from build123d import *

# Parameters (mm, degrees)
F1_DEPTH = 25.4


with BuildPart() as f1:
    # F0 (on Top) → F1 (new body)
    with BuildSketch(Plane.XY):
        with BuildLine():
            Line((-308.69023, -16.839156), (-308.69023, -82.879156))
            Line((-308.69023, -82.879156), (265.34977, -82.879156))
            Line((265.34977, -82.879156), (265.34977, -16.839156))
            Line((265.34977, -16.839156), (43.73477, -16.839156))
            ThreePointArc((43.73477, -16.839156), (11.405848, -3.448078), (-1.98523, 28.880844))
            Line((-1.98523, 28.880844), (-1.98523, 414.960844))
            ThreePointArc((-1.98523, 414.960844), (11.405848, 447.289766), (43.73477, 460.680844))
            Line((43.73477, 460.680844), (265.34977, 460.680844))
            Line((265.34977, 460.680844), (265.34977, 526.720844))
            Line((265.34977, 526.720844), (-308.69023, 526.720844))
            Line((-308.69023, 526.720844), (-308.69023, 460.680844))
            Line((-308.69023, 460.680844), (-87.07523, 460.680844))
            ThreePointArc((-87.07523, 460.680844), (-54.746308, 447.289766), (-41.35523, 414.960844))
            Line((-41.35523, 414.960844), (-41.35523, 301.353365))
            Line((-41.35523, 301.353365), (-41.35523, 28.880844))
            ThreePointArc((-41.35523, 28.880844), (-54.746308, -3.448078), (-87.07523, -16.839156))
            Line((-87.07523, -16.839156), (-308.69023, -16.839156))
        make_face()
    extrude(amount=F1_DEPTH)


solid = f1.part
Can you work these out from the model? Positions are in its coordinate system, mm. A direction names the side the tool comes from. Give positions to 0.01 mm unless a question says otherwise; leave off trailing zeros. Loops run counter-clockwise (first coordinate to the right, second up) from the corner with the lowest first, then second, coordinate; pieces in that order, holes last. Notation, with made-up numbers: M 30.5,5 L 86.5,5 A22 ccw 86.5,12 Z; hole C 34.5,66 d6. An arc over 180 degrees is marked long. One line per item, written item: value.
1) Imagine slicing it at B-B on z = 21. Write out the boundary of the cut face in (x, y), and give its area (3 significant figures).
Geometry check:
outline: M -308.69,-82.88 L 265.35,-82.88 L 265.35,-16.84 L 43.73,-16.84 A45.72 cw -1.99,28.88 L -1.99,414.96 A45.72 cw 43.73,460.68 L 265.35,460.68 L 265.35,526.72 L -308.69,526.72 L -308.69,460.68 L -87.08,460.68 A45.72 cw -41.36,414.96 L -41.36,28.88 A45.72 cw -87.08,-16.84 L -308.69,-16.84 Z
area: 96,400 mm²
2) Please list where these lines run through material, in increasing order: line 1 (Y direction, x = 67.5, z = 18.75); line 2 (X direction, y = 213, z = 4.75); line 3 (Y direction, x = 38.5, z = 23.5).
Geometry check:
line 1: y = -82.88 to -16.84, 460.68 to 526.72
line 2: x = -41.36 to -1.99
line 3: y = -82.88 to -16.54, 460.38 to 526.72
3) Imagine slicing it at C-C on x = -56. Write out the boundary of the cut face in (y, z).
Geometry check:
outline: M -82.88,0 L -4.65,0 L -4.65,25.4 L -82.88,25.4 Z; M 448.5,0 L 526.72,0 L 526.72,25.4 L 448.5,25.4 Z
4) I'm going to push a flat-ended pin straight in: pin 1 (1 mm diameter, centred on y = 263.5, z = 14.5, fed in from -X). Where does the tip first touch, or does it pass through?
Geometry check:
pin 1: stops at x = -41.36
5) Imagine slicing it at D-D on y = 337.5. Write out the boundary of the cut face in (x, z).
Geometry check:
outline: M -41.36,0 L -1.99,0 L -1.99,25.4 L -41.36,25.4 Z
6) On a 3-axis mill with a long thin cutter (end or side, diameter ignored), from which of +Z, -Z, +X, -X, +Y, -Y can I reach the whole of each face in a straight line? I mean faces 4 (the face through (-196, -16.839, 13)), 5 (the face through (-308.69, -49, 13)), 6 (the face through (11.05, 446.93, 12.52)). Say none if no direction works.
Geometry check:
face 4: +Z, -Z, -X
face 5: +Z, -Z, -X, +Y, -Y
face 6: +Z, -Z, +X
7) Thinking about a two-plate mould opening in Y: for faces 1 (the face through (-26, -82.879, 13)), 2 (the face through (-54.4, -3.1, 12.5)), 3 (the face through (-23, 201, 0)), which applies, +Y half, -Y half, draft (parallel to the pull), parting line (faces both ways), or undercut?
Geometry check:
face 1: -Y half
face 2: undercut
face 3: draft
8) Imagine slicing it at A-A on x = 198.5. Write out the boundary of the cut face in (y, z), and give its area (3 significant figures).
Geometry check:
outline: M -82.88,0 L -16.84,0 L -16.84,25.4 L -82.88,25.4 Z; M 460.68,0 L 526.72,0 L 526.72,25.4 L 460.68,25.4 Z
area: 3,350 mm²
